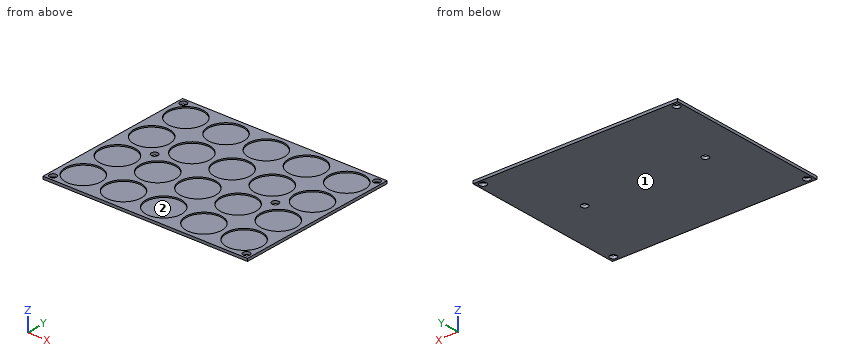
from build123d import *

# Parameters (mm, degrees)
F0_W     = 152.5
F0_H     = 122.5
F0_R     = 13.25
F1_DEPTH = 1
F2_DEPTH = 2
F3_R     = 2.55
F4_DEPTH = 2.001


# Not quite as in the source:
# - a feature names something its author has since deleted; it is built from what else it names


with BuildPart() as f1:
    # F0 (on Top) → F1 (new body)
    with BuildSketch(Plane.XY):
        Rectangle(F0_W, F0_H)
        with Locations((-60, -45)):
            Circle(F0_R, mode=Mode.SUBTRACT)
        with Locations((-30, -45)):
            Circle(F0_R, mode=Mode.SUBTRACT)
        with Locations((-60, -15)):
            Circle(F0_R, mode=Mode.SUBTRACT)
        with Locations((-30, -15)):
            Circle(F0_R, mode=Mode.SUBTRACT)
        with Locations((0, -45)):
            Circle(F0_R, mode=Mode.SUBTRACT)
        with Locations((30, -45)):
            Circle(F0_R, mode=Mode.SUBTRACT)
        with Locations((60, -45)):
            Circle(F0_R, mode=Mode.SUBTRACT)
        with Locations((0, -15)):
            Circle(F0_R, mode=Mode.SUBTRACT)
        with Locations((30, -15)):
            Circle(F0_R, mode=Mode.SUBTRACT)
        with Locations((60, -15)):
            Circle(F0_R, mode=Mode.SUBTRACT)
        with Locations((-60, 15)):
            Circle(F0_R, mode=Mode.SUBTRACT)
        with Locations((-30, 15)):
            Circle(F0_R, mode=Mode.SUBTRACT)
        with Locations((-60, 45)):
            Circle(F0_R, mode=Mode.SUBTRACT)
        with Locations((-30, 45)):
            Circle(F0_R, mode=Mode.SUBTRACT)
        with Locations((0, 15)):
            Circle(F0_R, mode=Mode.SUBTRACT)
        with Locations((30, 15)):
            Circle(F0_R, mode=Mode.SUBTRACT)
        with Locations((60, 15)):
            Circle(F0_R, mode=Mode.SUBTRACT)
        with Locations((0, 45)):
            Circle(F0_R, mode=Mode.SUBTRACT)
        with Locations((30, 45)):
            Circle(F0_R, mode=Mode.SUBTRACT)
        with Locations((60, 45)):
            Circle(F0_R, mode=Mode.SUBTRACT)
        with Locations((-60, 45)):
            Circle(F0_R)
        with Locations((-30, 45)):
            Circle(F0_R)
        with Locations((0, 45)):
            Circle(F0_R)
        with Locations((30, 45)):
            Circle(F0_R)
        with Locations((60, 45)):
            Circle(F0_R)
        with Locations((60, 15)):
            Circle(F0_R)
        with Locations((30, 15)):
            Circle(F0_R)
        with Locations((-30, 15)):
            Circle(F0_R)
        with Locations((-60, 15)):
            Circle(F0_R)
        with Locations((0, 15)):
            Circle(F0_R)
        with Locations((0, -15)):
            Circle(F0_R)
        with Locations((-30, -15)):
            Circle(F0_R)
        with Locations((-60, -15)):
            Circle(F0_R)
        with Locations((30, -15)):
            Circle(F0_R)
        with Locations((60, -15)):
            Circle(F0_R)
        with Locations((30, -45)):
            Circle(F0_R)
        with Locations((60, -45)):
            Circle(F0_R)
        with Locations((0, -45)):
            Circle(F0_R)
        with Locations((-30, -45)):
            Circle(F0_R)
        with Locations((-60, -45)):
            Circle(F0_R)
    extrude(amount=F1_DEPTH)

    # F0 (on Top) → F2 (join)
    with BuildSketch(Plane.XY):
        Rectangle(F0_W, F0_H)
        with Locations((-60, -45)):
            Circle(F0_R, mode=Mode.SUBTRACT)
        with Locations((-30, -45)):
            Circle(F0_R, mode=Mode.SUBTRACT)
        with Locations((-60, -15)):
            Circle(F0_R, mode=Mode.SUBTRACT)
        with Locations((-30, -15)):
            Circle(F0_R, mode=Mode.SUBTRACT)
        with Locations((0, -45)):
            Circle(F0_R, mode=Mode.SUBTRACT)
        with Locations((30, -45)):
            Circle(F0_R, mode=Mode.SUBTRACT)
        with Locations((60, -45)):
            Circle(F0_R, mode=Mode.SUBTRACT)
        with Locations((0, -15)):
            Circle(F0_R, mode=Mode.SUBTRACT)
        with Locations((30, -15)):
            Circle(F0_R, mode=Mode.SUBTRACT)
        with Locations((60, -15)):
            Circle(F0_R, mode=Mode.SUBTRACT)
        with Locations((-60, 15)):
            Circle(F0_R, mode=Mode.SUBTRACT)
        with Locations((-30, 15)):
            Circle(F0_R, mode=Mode.SUBTRACT)
        with Locations((-60, 45)):
            Circle(F0_R, mode=Mode.SUBTRACT)
        with Locations((-30, 45)):
            Circle(F0_R, mode=Mode.SUBTRACT)
        with Locations((0, 15)):
            Circle(F0_R, mode=Mode.SUBTRACT)
        with Locations((30, 15)):
            Circle(F0_R, mode=Mode.SUBTRACT)
        with Locations((60, 15)):
            Circle(F0_R, mode=Mode.SUBTRACT)
        with Locations((0, 45)):
            Circle(F0_R, mode=Mode.SUBTRACT)
        with Locations((30, 45)):
            Circle(F0_R, mode=Mode.SUBTRACT)
        with Locations((60, 45)):
            Circle(F0_R, mode=Mode.SUBTRACT)
    extrude(amount=F2_DEPTH)

    # F3 (on face) → F4 (cut, through all)
    with BuildSketch(Plane.XY.offset(2)):
        with Locations((-72.2, 57.2)):
            Circle(F3_R)
        with Locations((-45, 0)):
            Circle(F3_R)
        with Locations((72.2, 57.2)):
            Circle(F3_R)
        with Locations((45, 0)):
            Circle(F3_R)
        with Locations((72.2, -57.2)):
            Circle(F3_R)
        with Locations((-72.2, -57.2)):
            Circle(F3_R)
    extrude(amount=-F4_DEPTH, mode=Mode.SUBTRACT)


solid = f1.part
Geometry: final body of the model. Coordinates: model frame, mm. Face numbers are marked on the shaded views. Coordinates: 2 decimals unless noted, no trailing zeros. Loops run counter-clockwise (first coordinate to the right, second up) from the corner with the lowest first, then second, coordinate; pieces in that order, holes last. Notation, with made-up numbers: (7.5, -33.75) - (30.5, -33.75) arc R10 ccw to (30.5, -26.75) - close; hole circle Ø10 at (-32, 76.5). An arc over 180 degrees is marked (long way). Put each result on its own line as item: value. Start each with the question number.
Q1. Cut plane A-A, the plane z = 1.5. Give the number of separate pieces and of enclosed holes in the cut face, and give its area (3 significant figures).
Q2. Line query: line 1 (X direction, y = 45, z = 1.25); line 2 (Y direction, x = 0, z = 1.55); line 3 (X direction, y = 19, z = 1.45). Output: solid intervals per line, ascending.
Q3. Cut plane C-C, the plane y = 0. Return loops of the section in (x, z), and give its area (3 significant figures).
Q4. Cut plane D-D, the plane y = 45. Return loops of the section in (x, z), and give its area (4 significant figures).
Q5. Pin query (flat end, axial travel): pin 1 Ø24 at (x, y) = (-30, 45) entering from +Z; pin 2 Ø4.5 at (x, y) = (-72.2, 57.2) entering from -Z; pin 3 Ø8 at (x, y) = (-72.2, -57.2) entering from -Z. Return the tip coordinate at first contact, or that it passes through.
Q6. Cut plane B-B, the plane x = -45. Return loops of the section in (y, z).
Q7. Pull-direction query (Y, two-part tool) for the marked faces 1 and 2; classes: released by +Y, released by -Y, zero draft, split by the parting line, or undercut.
Filled sheet:
1. separate pieces: 1
1. enclosed holes: 26
1. area: 7,530 mm²
2. line 1: -76.25 to -73.25, -46.75 to -43.25, -16.75 to -13.25, 13.25 to 16.75, 43.25 to 46.75, 73.25 to 76.25
2. line 2: -61.25 to -58.25, -31.75 to -28.25, -1.75 to 1.75, 28.25 to 31.75, 58.25 to 61.25
2. line 3: -76.25 to -72.63, -47.37 to -42.63, -17.37 to -12.63, 12.63 to 17.37, 42.63 to 47.37, 72.63 to 76.25
3. outline: (-76.25, 0) - (-47.55, 0) - (-47.55, 2) - (-76.25, 2) - close; (-42.45, 0) - (42.45, 0) - (42.45, 2) - (-42.45, 2) - close; (47.55, 0) - (76.25, 0) - (76.25, 2) - (47.55, 2) - close
3. area: 285 mm²
4. outline: (-76.25, 0) - (76.25, 0) - (76.25, 2) - (73.25, 2) - (73.25, 1) - (46.75, 1) - (46.75, 2) - (43.25, 2) - (43.25, 1) - (16.75, 1) - (16.75, 2) - (13.25, 2) - (13.25, 1) - (-13.25, 1) - (-13.25, 2) - (-16.75, 2) - (-16.75, 1) - (-43.25, 1) - (-43.25, 2) - (-46.75, 2) - (-46.75, 1) - (-73.25, 1) - (-73.25, 2) - (-76.25, 2) - close
4. area: 172.5 mm²
5. pin 1: z = 1
5. pin 2: through
5. pin 3: z = 0
6. outline: (-61.25, 0) - (-2.55, 0) - (-2.55, 2) - (-61.25, 2) - close; (2.55, 0) - (61.25, 0) - (61.25, 2) - (2.55, 2) - close
7. face 1: zero draft
7. face 2: undercut
